Design review of the part built by this model. Coordinates are the model's own, in mm. A direction names the side the tool comes from. Round coordinates to 2 decimals unless told otherwise and drop trailing zeros. Order: outer loops, then holes, each group sorted by start corner. A loop starts at its lowest first (then second) coordinate and runs counter-clockwise, first axis right, second up. Notation, with made-up numbers: (58, -34.75) - (87, -34.75) arc R19 cw to (87, -22.75) - close; hole circle Ø10 at (67, 4). An arc over 180 degrees is marked (long way). Use CSV: the item, a comma, the result in double quotes. Start each with the question number.
from build123d import *

# Parameters (mm, degrees)
ESQUISSE1_W             = 12
ESQUISSE1_H             = 12
BOSS_EXTRU_1_DEPTH      = 4
ESQUISSE2_R             = 2
ENL_V_MAT_EXTRU_2_DEPTH = 4
ESQUISSE3_R             = 3.6
ENL_V_MAT_EXTRU_3_DEPTH = 2.5
ESQUISSE4_W             = 6
ESQUISSE4_H             = 4
BOSS_EXTRU_2_DEPTH      = 4
ESQUISSE5_R             = 1.25
BOSS_EXTRU_3_DEPTH      = 4
BOSS_EXTRU_3_TAPER      = 2
CHANFREIN1_SIZE2        = 0.5
CHANFREIN1_SIZE         = 0.518407978
CONG_1_R                = 0.3


with BuildPart() as part:
    # Esquisse1 → Boss.-Extru.1 (new body)
    with BuildSketch(Plane.XY):
        with Locations((6, 6)):
            Rectangle(ESQUISSE1_W, ESQUISSE1_H)
    extrude(amount=BOSS_EXTRU_1_DEPTH)

    # Esquisse2 → Enlèv. mat.-Extru.2 (cut)
    with BuildSketch(Plane.XY):
        with Locations((6, 6)):
            Circle(ESQUISSE2_R)
    extrude(amount=ENL_V_MAT_EXTRU_2_DEPTH, mode=Mode.SUBTRACT)

    # Esquisse3 → Enlèv. mat.-Extru.3 (cut)
    with BuildSketch(Plane.XY):
        with Locations((6, 6)):
            Circle(ESQUISSE3_R)
    extrude(amount=ENL_V_MAT_EXTRU_3_DEPTH, mode=Mode.SUBTRACT)

    # Esquisse4 → Boss.-Extru.2 (add)
    with BuildSketch(Plane.XY):
        with Locations((-3, 6)):
            Rectangle(ESQUISSE4_W, ESQUISSE4_H)
    extrude(amount=BOSS_EXTRU_2_DEPTH)

    # Esquisse5 → Boss.-Extru.3 (add)
    with BuildSketch(Plane.XY):
        with Locations((-4, 6)):
            Circle(ESQUISSE5_R)
    extrude(amount=-BOSS_EXTRU_3_DEPTH, taper=BOSS_EXTRU_3_TAPER)

    # Chanfrein1
    chanfrein1_edges = [part.edges().sort_by_distance(p)[0] for p in [
        (-5.110316922, 6, -4),
    ]]
    chamfer(chanfrein1_edges, length=CHANFREIN1_SIZE, length2=CHANFREIN1_SIZE2)

    # Congé1
    cong_1_edges = [part.edges().sort_by_distance(p)[0] for p in [
        (2.4, 6, 0),
        (0, 2, 0),
        (0, 4, 2),
        (-3, 8, 0),
        (-6, 6, 0),
        (-6, 8, 2),
        (-3, 4, 0),
        (-6, 4, 2),
        (-5.25, 6, 0),
        (6, 12, 0),
        (12, 6, 0),
        (6, 0, 0),
        (0, 10, 0),
        (0, 12, 2),
        (12, 12, 2),
        (12, 0, 2),
        (0, 0, 2),
    ]]
    fillet(cong_1_edges, radius=CONG_1_R)


solid = part.part
Q1. Take a section at A-A (z = 1.5). State the section outline as (x, y) points.
Q2. Take a section at B-B (x = 6). State the section outline as (y, z) points.
Q3. Take a section at C-C (x = -4). State the section outline as (y, z) points, plus the area to 3 significant figures.
Q4. Take a section at D-D (z = 3.5). State the section outline as (x, y) points.
Q5. Tool access review of faces 1 (the flat face through (0, 2, 2)), 2 (the flat face through (-3, 8, 2)), 3 (the flat face through (-4, 6, -4)), 4 (the cylindrical face through (7.935, 9.036, 1.385)): name each direction out of +Z, -Z, +X, -X, +Y, -Y from which nothing blocks a thin tool from reaching the whole face with its end or side.
Q6. Clearance check with flat-ended pins moving along their axes: pin 1 (3.5 mm diameter, centred on x = 7.5, y = 6.5, fed in from -Z); pin 2 (1 mm diameter, centred on y = 2.5, z = 3, fed in from -X); pin 3 (4 mm diameter, centred on x = -2.5, z = 2, fed in from -Y); pin 4 (2 mm diameter, centred on x = 4, z = -0.5, fed in from +Y). State where each tip first meets the part, or that it passes through.
Q7. For L1, parallel to Y at x = 6, z = 1.2; L2, parallel to Y at x = 6, z = 3.4; L3, parallel to Y at x = -1.5, z = 2.75, list the stretches that pass through material, from the lowest coordinate up. Write a range as [from, to].
Q8. The part is to be moulded in two halves that separate along X. For faces 5 (the flat face through (12, 6, 2)), 6 (the flat face through (8, 4, 2.5)), 7 (the cylindrical face through (4.526, 7.352, 3.24)), 8 (the flat face through (3, 6, 4)), say which applies: +X half, -X half, draft (parallel to the pull), parting line (faces both ways), or undercut.
Findings below:
1,outline,"(-6, 4.3) arc R0.3 ccw to (-5.7, 4) - (-0.3, 4) arc R0.3 cw to (0, 3.7) - (0, 0.3) arc R0.3 ccw to (0.3, 0) - (11.7, 0) arc R0.3 ccw to (12, 0.3) - (12, 11.7) arc R0.3 ccw to (11.7, 12) - (0.3, 12) arc R0.3 ccw to (0, 11.7) - (0, 8) - (-5.7, 8) arc R0.3 ccw to (-6, 7.7) - close; hole circle Ø7.2 at (6, 6)"
2,outline,"(0, 0.3) arc R0.3 ccw to (0.3, 0) - (2.1, 0) arc R0.3 ccw to (2.4, 0.3) - (2.4, 2.5) - (4, 2.5) - (4, 4) - (0, 4) - close; (8, 2.5) - (9.6, 2.5) - (9.6, 0.3) arc R0.3 ccw to (9.9, 0) - (11.7, 0) arc R0.3 ccw to (12, 0.3) - (12, 4) - (8, 4) - close"
3,outline,"(4, 0.3) arc R0.3 ccw to (4.3, 0) - (4.46, 0) arc R0.3 cw to (4.76, -0.29) - (4.87, -3.48) - (5.39, -4) - (6.61, -4) - (7.13, -3.48) - (7.24, -0.29) arc R0.3 cw to (7.54, 0) - (7.7, 0) arc R0.3 ccw to (8, 0.3) - (8, 4) - (4, 4) - close"
3,area,"25.2 mm^2"
4,outline,"(-6, 4.3) arc R0.3 ccw to (-5.7, 4) - (-0.3, 4) arc R0.3 cw to (0, 3.7) - (0, 0.3) arc R0.3 ccw to (0.3, 0) - (11.7, 0) arc R0.3 ccw to (12, 0.3) - (12, 11.7) arc R0.3 ccw to (11.7, 12) - (0.3, 12) arc R0.3 ccw to (0, 11.7) - (0, 8) - (-5.7, 8) arc R0.3 ccw to (-6, 7.7) - close; hole circle Ø4 at (6, 6)"
5,face 1,"+Z, -Z, -X, -Y"
5,face 2,"+Z, -Z, -X, +Y"
5,face 3,"-Z, +X, -X, +Y, -Y"
5,face 4,"-Z"
6,pin 1,"stops at z = 2.5"
6,pin 2,"stops at x = 0"
6,pin 3,"stops at y = 4"
6,pin 4,"stops at y = 12"
7,L1,"y = [0, 2.4], [9.6, 12]"
7,L2,"y = [0, 4], [8, 12]"
7,L3,"y = [4, 8]"
8,face 5,"+X half"
8,face 6,"undercut"
8,face 7,"undercut"
8,face 8,"draft"
